Geometry: final body of the model. Coordinates: model frame, mm. A direction names the side the tool comes from. Coordinates: 2 decimals unless noted, no trailing zeros. Loops run counter-clockwise (first coordinate to the right, second up) from the corner with the lowest first, then second, coordinate; pieces in that order, holes last. Notation, with made-up numbers: (-3.5, -31.75) -> (1.5, -31.75) arc R25 cw to (1.5, -15.75) -> close; hole circle Ø11 at (19, 60.5). An arc over 180 degrees is marked (long way). One line per item, written item: value. Start each with the question number.
Item 1: Ray query, probe 1 along X at (y, z) = (12.5, -11.5); probe 2 along Z at (x, y) = (233, -5); probe 3 along Y at (x, z) = (218.5, -3). Return the intervals inside material, ascending. Write a range as from..to.
Item 2: Section query D-D on y = 0. Return loops of the section in (x, z), then the cut area to 4 significant figures.
Item 3: Contact query for flat-ended pins moving along their axis: pin 1 Ø8 at (x, z) = (216, 0.5) entering from +Y; pin 2 Ø6 at (x, y) = (216.5, 11.5) entering from +Z; pin 3 Ø10 at (x, z) = (282.5, -10.5) entering from -Y. Output: stop coordinate, or through.
Item 4: Section query C-C on x = 188. Return loops of the section in (y, z), then the cut area to 3 significant figures.
Item 5: Set-up query: faces 1 (the flat face through (150.27, 9.57, 5.42)), 2 (the flat face through (304.8, 0, 12)), 3 (the flat face through (150.27, -9.57, -5.42)), 4 (the flat face through (150.27, 9.48, -5.58)). Return all of +Z, -Z, +X, -X, +Y, -Y with unobstructed straight access to the full face (end or side cutting, diameter ignored); none if empty.
Item 6: Section query A-A on z = -17. Return loops of the section in (x, y).
Item 7: Mould query, pull axis X, two halves, no side actions, for faces 5 (the flat face through (150, 0, 10.999)), 6 (the flat face through (-12.7, 0, 0)), 7 (the cylindrical face through (311.061, -5.506, -24.796)), 8 (the flat face through (317.5, 0, 0)). Classes: +X half, -X half, draft (parallel to the pull), parting line (faces both ways), or undercut.
Item 8: Section query B-B on y = 16.5. Return loops of the section in (x, z).
from build123d import *

# Parameters (mm, degrees)
F1_DEPTH = 304.8
F2_R     = 25.4
F3_DEPTH = 12.7
F4_R     = 25.4
F5_DEPTH = 12.7


with BuildPart() as f1:
    # F0 (on Right) → F1 (new body)
    with BuildSketch(Plane.YZ):
        Polygon((6.35, -10.9985226281), (12.7, 0), (6.35, 10.9985226281), (-6.35, 10.9985226281), (-12.7, 0), (-6.35, -10.9985226281), align=None)
    extrude(amount=F1_DEPTH)

    # F2 (on face) → F3 (join)
    with BuildSketch(Plane.YZ.offset(304.8)):
        Circle(F2_R)
        Polygon((6.35, -10.9985226281), (-6.35, -10.9985226281), (-12.7, 0), (-6.35, 10.9985226281), (6.35, 10.9985226281), (12.7, 0), align=None, mode=Mode.SUBTRACT)
        Polygon((-12.7, 0), (-6.35, -10.9985226281), (6.35, -10.9985226281), (12.7, 0), (6.35, 10.9985226281), (-6.35, 10.9985226281), align=None)
    extrude(amount=F3_DEPTH)

    # F4 (on face) → F5 (join)
    with BuildSketch(Plane(origin=(0, 0, 0), x_dir=(0, -1, 0), z_dir=(-1, 0, 0))):
        Circle(F4_R)
        Polygon((6.35, -10.9985226281), (-6.35, -10.9985226281), (-12.7, 0), (-6.35, 10.9985226281), (6.35, 10.9985226281), (12.7, 0), align=None, mode=Mode.SUBTRACT)
        Polygon((-12.7, 0), (-6.35, -10.9985226281), (6.35, -10.9985226281), (12.7, 0), (6.35, 10.9985226281), (-6.35, 10.9985226281), align=None)
    extrude(amount=F5_DEPTH)


solid = f1.part
Reply:
1. probe 1: x = -12.7..0, 304.8..317.5
1. probe 2: z = -11..11
1. probe 3: y = -10.97..10.97
2. outline: (-12.7, -25.4) -> (0, -25.4) -> (0, -11) -> (304.8, -11) -> (304.8, -25.4) -> (317.5, -25.4) -> (317.5, 25.4) -> (304.8, 25.4) -> (304.8, 11) -> (0, 11) -> (0, 25.4) -> (-12.7, 25.4) -> close
2. area: 7,995 mm²
3. pin 1: stops at y = 12.7
3. pin 2: stops at z = 7.27
3. pin 3: stops at y = -9.52
4. outline: (-12.7, 0) -> (-6.35, -11) -> (6.35, -11) -> (12.7, 0) -> (6.35, 11) -> (-6.35, 11) -> close
4. area: 419 mm²
5. face 1: +Z, +Y
5. face 2: none
5. face 3: -Z, -Y
5. face 4: -Z, +Y
6. outline: (-12.7, -18.87) -> (0, -18.87) -> (0, 18.87) -> (-12.7, 18.87) -> close; (304.8, -18.87) -> (317.5, -18.87) -> (317.5, 18.87) -> (304.8, 18.87) -> close
7. face 5: undercut
7. face 6: -X half
7. face 7: draft
7. face 8: +X half
8. outline: (-12.7, -19.31) -> (0, -19.31) -> (0, 19.31) -> (-12.7, 19.31) -> close; (304.8, -19.31) -> (317.5, -19.31) -> (317.5, 19.31) -> (304.8, 19.31) -> close
